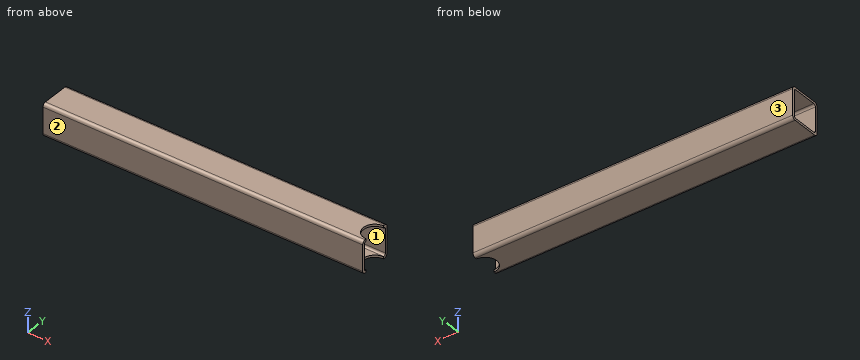
```python
from build123d import *

# Parameters (mm, degrees)
EXTRUDE_1_DEPTH = 297.016771071
OTHER_START     = -15
OTHER_1_DEPTH   = 30


# Read off the part's stored shape, not the designer's step: Полость1
with BuildPart() as part:
    # Эскиз1 → Бобышка-Вытянуть1 (new body)
    with BuildSketch(Plane(origin=(0, 0, 0), x_dir=(0, 0, -1), z_dir=(1, 0, 0))):
        with BuildLine():
            Line((-12, 15), (12, 15))
            ThreePointArc((12, 15), (14.121320344, 14.121320344), (15, 12))
            Line((15, 12), (15, -12))
            ThreePointArc((15, -12), (14.121320344, -14.121320344), (12, -15))
            Line((12, -15), (-12, -15))
            ThreePointArc((-12, -15), (-14.121320344, -14.121320344), (-15, -12))
            Line((-15, -12), (-15, 12))
            ThreePointArc((-15, 12), (-14.121320344, 14.121320344), (-12, 15))
        make_face()
        with BuildLine():
            Line((-11, 13), (11, 13))
            ThreePointArc((11, 13), (12.414213562, 12.414213562), (13, 11))
            Line((13, 11), (13, -11))
            ThreePointArc((13, -11), (12.414213562, -12.414213562), (11, -13))
            Line((11, -13), (-11, -13))
            ThreePointArc((-11, -13), (-12.414213562, -12.414213562), (-13, -11))
            Line((-13, -11), (-13, 11))
            ThreePointArc((-13, 11), (-12.414213562, 12.414213562), (-11, 13))
        make_face(mode=Mode.SUBTRACT)
    extrude(amount=-EXTRUDE_1_DEPTH)

    # Полость1 outline → Полость1 (cut)
    with BuildSketch(Plane.XY.offset(OTHER_START)):
        with BuildLine():
            Line((0, -10.65), (0, 10.65))
            ThreePointArc((0, 10.65), (-10.65, 0), (0, -10.65))
        make_face()
    extrude(amount=OTHER_1_DEPTH, mode=Mode.SUBTRACT)


solid = part.part
```
Source: CAD feature listing. Evaluate the final solid. Frame: model axes, mm. Face numbers are marked on the shaded views. Give positions to 0.01 mm unless a question says otherwise; leave off trailing zeros. Write each loop counter-clockwise with the first axis right and the second up, starting at its lowest first coordinate (ties: lowest second). Pieces come first, ordered by that corner, then holes.
1. Section query B-B (z = -7). Return the cut outline in (x, y).
2. Material intervals for line 1 along Z through (x, y) = (-230.5, -5); line 2 along Y through (x, z) = (-24, 13.5), sorted ascending.
3. Section query C-C (x = -74.5). Return the cut outline in (y, z).
4. Pull-direction query (Y, two-part tool) for the marked faces 1, 2 and 3; classes: +Y half, -Y half, draft (parallel to the pull), parting line (faces both ways), or undercut.
5. Section query A-A (y = 0). Return the cut outline in (x, z), then the cut area to 3 significant figures.
6. First-contact query: pin 1 (10 mm diameter, centred on y = 4, z = -2.5, fed in from +X). Flat tip, straight axial feed; report the tip coordinate or a pass-through.
Output values:
1. outline: (-297.02, -15) - (0, -15) - (0, -13) - (-297.02, -13) - close; (-297.02, 13) - (0, 13) - (0, 15) - (-297.02, 15) - close
2. line 1: z = -15 to -13, 13 to 15
2. line 2: y = -14.6 to 14.6
3. outline: (-15, -12) arc R3 ccw to (-12, -15) - (12, -15) arc R3 ccw to (15, -12) - (15, 12) arc R3 ccw to (12, 15) - (-12, 15) arc R3 ccw to (-15, 12) - close; hole (-13, -11) arc R2 ccw to (-11, -13) - (11, -13) arc R2 ccw to (13, -11) - (13, 11) arc R2 ccw to (11, 13) - (-11, 13) arc R2 ccw to (-13, 11) - close
4. face 1: undercut
4. face 2: -Y half
4. face 3: +Y half
5. outline: (-297.02, -15) - (-10.65, -15) - (-10.65, -13) - (-297.02, -13) - close; (-297.02, 13) - (-10.65, 13) - (-10.65, 15) - (-297.02, 15) - close
5. area: 1,150 mm2
6. pin 1: passes through
